Geometry: final body of the model. Coordinates: model frame, mm. Face numbers are marked on the shaded views. A direction names the side the tool comes from. Give positions to 0.01 mm unless a question says otherwise; leave off trailing zeros. Write each loop counter-clockwise with the first axis right and the second up, starting at its lowest first coordinate (ties: lowest second). Pieces come first, ordered by that corner, then holes. Notation, with made-up numbers: (3, 60.5) - (26, 60.5) arc R38 cw to (26, 98.5) - close; hole circle Ø5 at (81.5, -10). An arc over 180 degrees is marked (long way). Return JSON: item names as keys, results as strings.
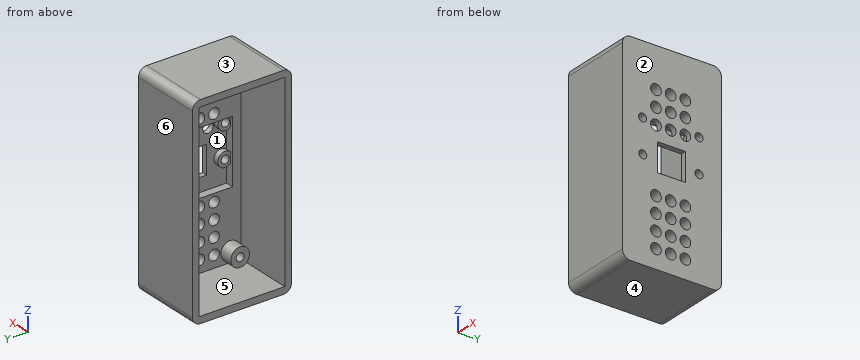
Autodesk Fusion 360 part; units mm, degrees
sketch "main_shape" plane through (-3, 0, 0) normal (-1, 0, 0) x (0, -1, 0)
  line L0 (-16, -35.5) -> (16, -35.5)
  line L1 (16, -35.5) -> (16, 35.5)
  line L2 (16, 35.5) -> (-16, 35.5)
  line L3 (-16, 35.5) -> (-16, -35.5)
  line L4 (-16, -35.5) -> (16, 35.5) construction
  line L5 (16, -35.5) -> (-16, 35.5) construction
  line L6 (-12, -41.3396) -> (-12, 39)
  line L7 (37, 0) -> (-27, 0)
  line L8 (37, 31.5) -> (-27, 31.5)
  circle A0 centre (-12, 31.5) radius 1.5
  circle A1 centre (-12, -31.5) radius 1.5
  line L9 (0, 42) -> (0, -40.4906)
  circle A2 centre (12, 31.5) radius 1.5
  circle A3 centre (12, -31.5) radius 1.5
  line L10 (18.5, -38) -> (18.5, 38)
  line L11 (18.5, 38) -> (-18.5, 38)
  line L12 (-18.5, 38) -> (-18.5, -38)
  line L13 (-18.5, -38) -> (18.5, -38)
  spline S0 degree 3 poles (44.3606, -31.4828) (42.7106, -31.4828) (41.3606, -30.1328) (41.3606, -28.4828) knots 1 1 1 1 2 2 2 2
  circle A4 centre (67.7694, -28.0995) radius 1.4
  circle A5 centre (44.7721, -28.0995) radius 1.4
  line L14 (68.3606, -31.4828) -> (44.3606, -31.4828)
  spline S1 degree 3 poles (71.3606, -28.4828) (71.3606, -30.1328) (70.0106, -31.4828) (68.3606, -31.4828) knots 7 7 7 7 8 8 8 8
  line L15 (0.4061, -10.074) -> (-12.0849, -10.074)
  line L16 (41.3606, -28.4828) -> (41.3606, 30.5172)
  line L17 (71.3606, 30.5172) -> (71.3606, -28.4828)
  line L18 (-12.0849, 13.92) -> (12.9147, 13.92)
  line L19 (44.3606, 33.5172) -> (68.3606, 33.5172)
  line L20 (12.9147, -10.074) -> (0.4061, -10.074)
  line L21 (5.4993, -4.9973) -> (-5.0007, -4.9956)
  line L22 (-4.999, 5.5044) -> (5.501, 5.5027)
  line L23 (50.5, -120.5) -> (65.5, -120.5)
  line L24 (65.5, -120.5) -> (65.5, -105.5)
  circle A6 centre (-10.0913, 11.9264) radius 1.5
  line L25 (5.501, 5.5027) -> (5.4993, -4.9973)
  line L26 (5.501, 5.5027) -> (-5.0007, -4.9956) construction
  circle A7 centre (10.9961, 11.9264) radius 1.5
  circle A8 centre (58, -113) radius 4
  line L27 (5.4993, -4.9973) -> (-4.999, 5.5044) construction
  line L28 (-5.0007, -4.9956) -> (-4.999, 5.5044)
  spline S2 degree 3 poles (41.3606, 30.5172) (41.3606, 32.1672) (42.7106, 33.5172) (44.3606, 33.5172) knots 3 3 3 3 4 4 4 4
  line L29 (-12.0849, -10.074) -> (-12.0849, 13.92)
  circle A9 centre (67.7694, 29.8978) radius 1.4
  circle A10 centre (-10.0913, -0.5652) radius 1.5
  circle A11 centre (44.7718, 29.8978) radius 1.4
  line L30 (64.5, -119.5) -> (51.5, -119.5)
  spline S3 degree 3 poles (68.3606, 33.5172) (70.0106, 33.5172) (71.3606, 32.1672) (71.3606, 30.5172) knots 5 5 5 5 6 6 6 6
  line L31 (51.5, -119.5) -> (64.5, -106.5) construction
  line L32 (50.5, -105.5) -> (50.5, -120.5)
  line L33 (65.5, -105.5) -> (50.5, -105.5)
  line L34 (64.5, -119.5) -> (51.5, -106.5) construction
  line L35 (65.5, -120.5) -> (50.5, -105.5) construction
  line L36 (12.9147, 13.92) -> (12.9147, -10.074)
  line L37 (52, -119) -> (64, -107) construction
  line L38 (64, -119) -> (52, -107) construction
  line L39 (51.5, -119.5) -> (51.5, -106.5)
  line L40 (50.5, -120.5) -> (65.5, -105.5) construction
  line L41 (51.5, -106.5) -> (64.5, -106.5)
  line L42 (64.5, -106.5) -> (64.5, -119.5)
  circle A12 centre (10.9211, -0.5307) radius 1.5
  circle A13 centre (12, 31.5) radius 3.5
  circle A14 centre (-12, 31.5) radius 3.5
  circle A15 centre (12, -31.5) radius 3.5
  circle A16 centre (-12, -31.5) radius 3.5
  circle A17 centre (0.5, -1) radius 2
  circle A18 centre (-5, 23) radius 2
  circle A19 centre (0.5, 23) radius 2
  circle A20 centre (6, 23) radius 2
  circle A21 centre (-5, 17) radius 2
  circle A22 centre (0.5, 17) radius 2
  circle A23 centre (6, 17) radius 2
  circle A24 centre (-5, 11) radius 2
  circle A25 centre (0.5, 11) radius 2
  circle A26 centre (6, 11) radius 2
  circle A27 centre (-5, 5) radius 2
  circle A28 centre (0.5, 5) radius 2
  circle A29 centre (6, 5) radius 2
  circle A30 centre (-5, -1) radius 2
  circle A31 centre (6, -1) radius 2
  circle A32 centre (10.9961, 11.9264) radius 2.75
  circle A33 centre (-10.0913, 11.9264) radius 2.75
  circle A34 centre (-10.0913, -0.5652) radius 2.75
  circle A35 centre (10.9211, -0.5307) radius 2.75
  circle A36 centre (-5, -7) radius 2
  circle A37 centre (0.5, -7) radius 2
  circle A38 centre (6, -7) radius 2
  circle A39 centre (-5, -13) radius 2
  circle A40 centre (0.5, -13) radius 2
  circle A41 centre (6, -13) radius 2
  circle A42 centre (-5, -19) radius 2
  circle A43 centre (0.5, -19) radius 2
  circle A44 centre (6, -19) radius 2
  circle A45 centre (-5, -25) radius 2
  circle A46 centre (0.5, -25) radius 2
  circle A47 centre (6, -25) radius 2
  circle A48 centre (-5, -31) radius 2
  circle A49 centre (0.5, -31) radius 2
  circle A50 centre (6, -31) radius 2
  point P0 (-8, 0)
  point P1 (58, -113)
  point P2 (0.2502, 0.2536)
  point P3 (58, -113)
  point P4 (58, -113)
  dimension "d80" = 32
  dimension "d81" = 71
  dimension "d84" = 31.5
  dimension "d85" = 3
  dimension "d86" = 2.5
  dimension "d103" = 12
  dimension "d104" = 15
  dimension "d105" = 8
  dimension "d106" = 13
  dimension "d107" = 13
  dimension "d108" = 10.5
  dimension "d109" = 10.5
  dimension "d110" = 3
  dimension "d111" = 3
  dimension "d112" = 3
  dimension "d113" = 3
  dimension "d114" = 7
  dimension "d115" = 7
  dimension "d116" = 7
  dimension "d129" = 4
  dimension "d132" = 5.5
  dimension "d133" = -30
  dimension "d138" = 5.5
  dimension "d139" = 5.5
  dimension "d140" = 5.5
  dimension "d141" = 5.5
extrude "Extrude23" add sketch "main_shape" against normal blind 2 contours L0 L3 L6 L7 L15 L29 A16 A34 | L0 L3 L6 L7 L12 L13 | L0 L6 L9 L15 A16 A40 A43 A46 A49 | L0 L6 L9 L13 | L3 L7 L8 L12 | L3 L6 L7 L8 L18 L29 A14 A33 A34 | L0 L1 L7 L9 L15 L20 L36 A35 A40 A43 A46 A49 | L0 L1 L7 L9 L10 L13 | L6 A1 A16 | L6 A1 A16 | L2 L3 L6 L8 L11 L12 | L2 L3 L6 L8 A14 | L7 L29 A34 | L7 L29 A34 | L9 A49 | L9 A49 | L6 A1 | L6 A1 | L6 L8 A0 A14 | L6 L8 A0 A14 | L6 L7 L29 A34 | L6 L7 L29 A34 | L6 L29 A33 A34 | L6 L15 L29 A34 | L1 L7 L8 L9 L18 L36 A13 A19 A22 A32 A35 | L1 L7 L8 L10 | L6 L7 L9 L15 L21 L28 A30 A34 A37 | L2 L6 L9 L11 | L2 L6 L8 L9 A14 | L6 L8 A0 | L6 L8 A0 | L6 L8 A0 A14 | L6 L8 L9 L18 A14 A19 A22 A33 | L6 L8 A0 A14 | L6 L7 A10 A34 | L6 L7 A10 A34 | L29 A33 | L6 L29 A33 | L6 L7 L9 L18 L22 L28 A25 A27 A28 A30 A33 A34 | L1 L2 L8 L9 A13 | L1 L2 L8 L9 L10 L11 | L7 L36 A35 | L7 L36 A35 | L9 A46 | L9 A46 | L7 L9 L15 L20 L21 L25 L36 A31 A35 A37 | L6 L8 A0 | L6 L8 A0 | L6 L18 A33 | L6 L18 L29 A33 | L7 A10 | L6 L18 A33 | L8 A2 A13 | L8 A2 A13 | L7 L36 A12 A35 | L7 L36 A12 A35 | L7 L9 L18 L22 L25 L36 A25 A28 A29 A31 A32 A35 | L9 A37 | L9 A37 | L9 A40 | L9 A40 | L18 A33 | L7 L28 A30 | L7 L28 A30 | L8 A2 | L8 A2 | L7 A12 | L18 L36 A32 | L36 A32 | L9 A43 | L9 A43 | L9 A19 | L9 A19 | L18 L36 A32 | L18 A32 | L7 L25 A31 | L7 L25 A31 | L22 L28 A27 | L9 A22 | L9 A22 | L9 A25 | L9 A25 | L22 L25 A29 | L9 L22 A28 | L9 L22 A28 | A3 | A15 | A18 | A20 | A21 | A23 | A24 | A26 | A36 | A38 | A39 | A41 | A42 | A44 | A45 | A47 | A48 | A50 picked at (-10.5906, -0.2157) picked at (-5.0991, 0.6592) picked at (-5.0995, -1.9925) picked at (10.4334, -0.2871) picked at (6.4927, -1.8218) picked at (5.5949, 0.6416) picked at (-5.0979, 3.8421) picked at (7.1601, 5.2635) picked at (-0.5418, 6.1699) picked at (1.5934, 5.5934)
extrude "Extrude24" add sketch "main_shape" along normal blind 20 contours L0 L3 L6 L7 L12 L13 | L0 L6 L9 L13 | L3 L7 L8 L12 | L0 L1 L7 L9 L10 L13 | L2 L3 L6 L8 L11 L12 | L1 L7 L8 L10 | L2 L6 L9 L11 | L1 L2 L8 L9 L10 L11
extrude "Extrude25" add sketch "main_shape" along normal blind 8 contours L6 A1 A16 | L6 A1 A16 | L6 L8 A0 A14 | L6 L8 A0 A14 | L6 L8 A0 A14 | L6 L8 A0 A14 | L8 A2 A13 | L8 A2 A13 | A15
extrude "Extrude26" add sketch "main_shape" along normal blind 3 contours L0 L3 L6 L7 L15 L29 A16 A34 | L0 L6 L9 L15 A16 A40 A43 A46 A49 | L3 L6 L7 L8 L18 L29 A14 A33 A34 | L0 L1 L7 L9 L15 L20 L36 A35 A40 A43 A46 A49 | L2 L3 L6 L8 A14 | L7 L29 A34 | L7 L29 A34 | L9 A49 | L9 A49 | L1 L7 L8 L9 L18 L36 A13 A19 A22 A32 A35 | L2 L6 L8 L9 A14 | L6 L8 L9 L18 A14 A19 A22 A33 | L29 A33 | L1 L2 L8 L9 A13 | L7 L36 A35 | L7 L36 A35 | L9 A46 | L9 A46 | L9 A40 | L9 A40 | L18 A33 | L36 A32 | L9 A43 | L9 A43 | L9 A19 | L9 A19 | L18 A32 | L9 A22 | L9 A22 | A18 | A20 | A21 | A23 | A39 | A41 | A42 | A44 | A45 | A47 | A48 | A50
extrude "Extrude27" cut sketch "main_shape" against normal blind 14 contours L7 A10 | L7 A12 picked at (-10.5906, -0.2157) picked at (10.4334, -0.2871)
extrude "Extrude28" cut sketch "main_shape" along normal mid plane 36 contours L9 A49 | L9 A49 | L9 A46 | L9 A46 | L9 A40 | L9 A40 | L9 A43 | L9 A43 | L9 A19 | L9 A19 | L9 A22 | L9 A22 | L9 A25 | L9 A25 | A18 | A20 | A21 | A23 | A24 | A26 | A39 | A41 | A42 | A44 | A45 | A47 | A48 | A50
extrude "Extrude29" add 1 faces at (-23, -17.6667, -11.8333) along direction (-1, 0, 0) blind 5
extrude "Extrude30" add sketch "main_shape" along normal blind 2 contours L7 L29 A34 | L7 L29 A34 | L6 L7 L29 A34 | L6 L7 L29 A34 | L6 L7 A10 A34 | L6 L7 A10 A34 | L29 A33 | L7 L36 A35 | L7 L36 A35 | L6 L18 A33 | L7 L36 A12 A35 | L7 L36 A12 A35 | L18 A33 | L18 L36 A32 | L36 A32 | L18 A32 picked at (-10.0539, 13.754) picked at (11.0335, 13.754)
fillet "Fillet9" radius 3 1 edges at (-14.5, -18.5, -38)
fillet "Fillet10" radius 3 1 edges at (-14.5, 18.5, -38)
fillet "Fillet11" radius 3 2 edges at (-14.5, -18.5, 38) (-14.5, 18.5, 38)
equation "d84 = ( 63 / 2 ) * 1 mm"
Q1. Material intervals for probe 1 along Y at (x, z) = (-3.25, -13); probe 2 along Y at (x, z) = (-7, 11.5); probe 3 along Z at (x, y) = (-10, 3.5), sorted ascending. Write a range as [from, to].
Answer key:
{"probe 1": "y = [-18.5, -8], [-4, -2.5], [1.5, 3], [7, 18.5]", "probe 2": "y = [-18.5, -16], [16, 18.5]", "probe 3": "z = [-38, -35.5], [35.5, 38]"}
Q2. Pin query (flat end, axial travel): P1, Ø10, axis at y = -6, z = -24, coming from the -X side; P2, Ø4.5, axis at y = -0.5, z = 17, coming from the +X side; P3, Ø6.5, axis at y = -6, z = -31, coming from the -X side; P4, Ø7, axis at y = -3.5, z = 1.5, coming from the -X side. Return the tip coordinate at first contact, or that it passes through.
Answer key:
{"P1": "stops at x = -6", "P2": "stops at x = -1", "P3": "stops at x = -11", "P4": "stops at x = -3"}
Q3. Mould query, pull axis Z, two halves, no side actions, for the marked faces 1, 2, 3 and 4. Classes: pulls with the +Z half, pulls with the -Z half, needs draft (parallel to the pull), parting line crosses it, or undercut.
Answer key:
{"face 1": "undercut", "face 2": "needs draft", "face 3": "pulls with the +Z half", "face 4": "pulls with the -Z half"}
Q4. Section query B-B, the plane x = -22.75. Return the cut outline in (y, z), plus the area to 3 significant figures.
Answer key:
{"outline": "(-18.5, -35) arc R3 ccw to (-15.5, -38) - (15.5, -38) arc R3 ccw to (18.5, -35) - (18.5, 35) arc R3 ccw to (15.5, 38) - (-15.5, 38) arc R3 ccw to (-18.5, 35) - close; hole (-16, -35.5) - (16, -35.5) - (16, 35.5) - (-16, 35.5) - close", "area": "532 mm^2"}
Q5. Set-up query: the marked faces 5 and 6. Return all of +Z, -Z, +X, -X, +Y, -Y with unobstructed straight access to the full face (end or side cutting, diameter ignored); none if empty.
Answer key:
{"face 5": "-X", "face 6": "+Z, -Z, +X, -X, +Y"}
Q6. Section query D-D, the plane z = 4. Return the cut outline in (x, y).
Answer key:
{"outline": "(-28, -18.5) - (-1, -18.5) - (-1, -5.5) - (-3, -5.5) - (-3, -12.91) - (-6, -12.91) - (-6, -16) - (-28, -16) - close; (-28, 16) - (-6, 16) - (-6, 12.08) - (-3, 12.08) - (-3, 5) - (-1, 5) - (-1, 18.5) - (-28, 18.5) - close"}
Q7. Section query C-C, the plane z = 31.5. Return the cut outline in (x, y).
Answer key:
{"outline": "(-28, -18.5) - (-1, -18.5) - (-1, 18.5) - (-28, 18.5) - (-28, 16) - (-6, 16) - (-6, 15.5) - (-11, 15.5) - (-11, 13.5) - (-3, 13.5) - (-3, 10.5) - (-11, 10.5) - (-11, 8.5) - (-6, 8.5) - (-6, -8.5) - (-11, -8.5) - (-11, -10.5) - (-3, -10.5) - (-3, -13.5) - (-11, -13.5) - (-11, -15.5) - (-6, -15.5) - (-6, -16) - (-28, -16) - close"}
Q8. Section query A-A, the plane z = -25. Return the cut outline in (x, y), plus the area to 3 significant figures.
Answer key:
{"outline": "(-28, -18.5) - (-1, -18.5) - (-1, -8) - (-6, -8) - (-6, -16) - (-28, -16) - close; (-28, 16) - (-6, 16) - (-6, 7) - (-1, 7) - (-1, 18.5) - (-28, 18.5) - close; (-6, -4) - (-1, -4) - (-1, -2.5) - (-6, -2.5) - close; (-6, 1.5) - (-1, 1.5) - (-1, 3) - (-6, 3) - close", "area": "235 mm^2"}
